The model under review builds one solid part; all positions refer to its coordinate system, in mm. A direction names the side the tool comes from. Coordinates: 2 decimals unless noted, no trailing zeros. Order: outer loops, then holes, each group sorted by start corner. A loop starts at its lowest first (then second) coordinate and runs counter-clockwise, first axis right, second up. Notation, with made-up numbers: M 40.5,58 L 83.5,58 A14 cw 83.5,75 Z; hole C 21.25,10.5 d9. An arc over 180 degrees is marked long. Answer as CSV lines item,"result". Start each with the question number.
Q1. Machinability: for faces 4 (the face through (19.48, 9.86, 19.41)), 5 (the face through (-16.754, 4.93, 50.282)), 6 (the face through (18, 5, 53)), 7 (the face through (9, 15, 40)), 8 (the face through (-51.03, 4.93, -11.14)), which of the approach directions +Z, -Z, +X, -X, +Y, -Y give a long, thin tool a straight path to every point of the face, cutting with its end or side? Answer none if there is none.
Q2. Consider section B-B on z = 9. Write out the cut boundary in (x, y).
Q3. The part is to be moulded in two halves that separate along Z. For faces 1 (the face through (43.39, 4.93, -49.58)), 2 (the face through (-56.438, 4.93, 47.596)), 3 (the face through (27.737, 9.86, 15.957)), say which applies: +Z half, -Z half, draft (parallel to the pull), parting line (faces both ways), or undercut.
Q4. Wall thickness on L1, parallel to Z at x = 35, y = 8.25; L2, parallel to Z at x = 9.5, y = 4; L3, parallel to Y at x = -41, z = 38: over which ranges is each line inside the solid? List them lowest first. Write a range as [from, to].
Q5. For P1, Ø2.5, axis at y = 13.5, z = -30.5, coming from the -X side; P2, Ø2.5, axis at y = 10.5, z = -30, coming from the +X side; P3, Ø10, axis at x = -36, z = -30, coming from the +Y side; P4, Ø3.5, axis at y = 12, z = 30.5, coming from the -X side, all flat-tipped, find the tip position at first contact; note any pin that passes through.
Q6. Consider section A-A on x = -65. Write out the cut boundary in (y, z).
Q7. Consider section C-C on z = -23.5. Write out the cut boundary in (x, y), and give its area (3 significant figures).
Autodesk Inventor part; units mm, degrees
ref_plane "YZ Plane" through (0, 0, 0) normal (1, 0, 0) x (0, 1, 0)
ref_plane "XZ Plane" through (0, 0, 0) normal (0, 1, 0) x (-1, 0, 0)
ref_plane "XY Plane" through (0, 0, 0) normal (0, 0, 1) x (1, 0, 0)
sketch "Sketch1" plane through (0, 0, 0) normal (0, 1, 0) x (-1, 0, 0)
  circle A0 centre (0, 0) radius 41
  line L0 (-47, 0) -> (-47, 41)
  line L1 (-35, 53) -> (0, 53)
  circle A1 centre (-35, 41) radius 6
  arc A2 (-35, 53) -> (-47, 41) centre (-35, 41) ccw
  circle A3 centre (73.6122, 42.5) radius 6
  circle A4 centre (56.2917, 32.5) radius 6
  line L2 (0, 0) -> (41, 0) construction
  line L3 (0, 0) -> (35.507, 20.5) construction
  line L4 (35.507, 20.5) -> (56.2917, 32.5) construction
  line L5 (56.2917, 32.5) -> (73.6122, 42.5) construction
  arc A5 (80.1122, 31.2417) -> (67.1122, 53.7583) centre (73.6122, 42.5) ccw
  line L6 (67.1122, 53.7583) -> (45.4615, 41.2583)
  line L7 (80.1122, 31.2417) -> (59, 19.0526)
  arc A6 (59, 19.0526) -> (48, 0) centre (70, 0) ccw
  arc A7 (32.1763, 42.1151) -> (45.4615, 41.2583) centre (39.4615, 51.6506) ccw
  line L8 (41, 0) -> (48, 0) construction
  circle A8 centre (73.6122, -42.5) radius 6
  circle A9 centre (56.2917, -32.5) radius 6
  arc A10 (67.1122, -53.7583) -> (80.1122, -31.2417) centre (73.6122, -42.5) ccw
  line L9 (67.1122, -53.7583) -> (45.4615, -41.2583)
  line L10 (80.1122, -31.2417) -> (59, -19.0526)
  arc A11 (48, 0) -> (59, -19.0526) centre (70, 0) ccw
  arc A12 (45.4615, -41.2583) -> (32.1763, -42.1151) centre (39.4615, -51.6506) ccw
  arc A13 (3.5, 31.808) -> (-3.5, 31.808) centre (0, 0) ccw
  arc A14 (10.6071, 25.372) -> (3.5, 27.2764) centre (0, 0) ccw
  line L11 (3.5, 31.808) -> (3.5, 27.2764)
  arc A15 (-12.8729, 29.2966) -> (-18.9351, 25.7966) centre (0, 0) ccw
  line L12 (-12.8729, 29.2966) -> (-10.6071, 25.372)
  arc A16 (-25.7966, 18.9351) -> (-29.2966, 12.8729) centre (0, 0) ccw
  line L13 (-25.7966, 18.9351) -> (-21.872, 16.6693)
  arc A17 (-31.808, 3.5) -> (-31.808, -3.5) centre (0, 0) ccw
  line L14 (-31.808, 3.5) -> (-27.2764, 3.5)
  arc A18 (-29.2966, -12.8729) -> (-25.7966, -18.9351) centre (0, 0) ccw
  line L15 (-29.2966, -12.8729) -> (-25.372, -10.6071)
  arc A19 (-18.9351, -25.7966) -> (-12.8729, -29.2966) centre (0, 0) ccw
  line L16 (-18.9351, -25.7966) -> (-16.6693, -21.872)
  arc A20 (-3.5, -31.808) -> (3.5, -31.808) centre (0, 0) ccw
  line L17 (-3.5, -31.808) -> (-3.5, -27.2764)
  arc A21 (12.8729, -29.2966) -> (18.9351, -25.7966) centre (0, 0) ccw
  line L18 (12.8729, -29.2966) -> (10.6071, -25.372)
  arc A22 (25.7966, -18.9351) -> (29.2966, -12.8729) centre (0, 0) ccw
  line L19 (25.7966, -18.9351) -> (21.872, -16.6693)
  arc A23 (31.808, -3.5) -> (31.808, 3.5) centre (0, 0) ccw
  line L20 (31.808, -3.5) -> (27.2764, -3.5)
  arc A24 (29.2966, 12.8729) -> (25.7966, 18.9351) centre (0, 0) ccw
  line L21 (29.2966, 12.8729) -> (25.372, 10.6071)
  arc A25 (18.9351, 25.7966) -> (12.8729, 29.2966) centre (0, 0) ccw
  line L22 (18.9351, 25.7966) -> (16.6693, 21.872)
  line L23 (10.6071, 25.372) -> (12.8729, 29.2966)
  arc A26 (-3.5, 27.2764) -> (-10.6071, 25.372) centre (0, 0) ccw
  line L24 (-3.5, 27.2764) -> (-3.5, 31.808)
  arc A27 (-16.6693, 21.872) -> (-21.872, 16.6693) centre (0, 0) ccw
  line L25 (-16.6693, 21.872) -> (-18.9351, 25.7966)
  arc A28 (-25.372, 10.6071) -> (-27.2764, 3.5) centre (0, 0) ccw
  line L26 (-25.372, 10.6071) -> (-29.2966, 12.8729)
  arc A29 (-27.2764, -3.5) -> (-25.372, -10.6071) centre (0, 0) ccw
  line L27 (-27.2764, -3.5) -> (-31.808, -3.5)
  arc A30 (-21.872, -16.6693) -> (-16.6693, -21.872) centre (0, 0) ccw
  line L28 (-21.872, -16.6693) -> (-25.7966, -18.9351)
  arc A31 (-10.6071, -25.372) -> (-3.5, -27.2764) centre (0, 0) ccw
  line L29 (-10.6071, -25.372) -> (-12.8729, -29.2966)
  arc A32 (3.5, -27.2764) -> (10.6071, -25.372) centre (0, 0) ccw
  line L30 (3.5, -27.2764) -> (3.5, -31.808)
  arc A33 (16.6693, -21.872) -> (21.872, -16.6693) centre (0, 0) ccw
  line L31 (16.6693, -21.872) -> (18.9351, -25.7966)
  arc A34 (25.372, -10.6071) -> (27.2764, -3.5) centre (0, 0) ccw
  line L32 (25.372, -10.6071) -> (29.2966, -12.8729)
  arc A35 (27.2764, 3.5) -> (25.372, 10.6071) centre (0, 0) ccw
  line L33 (27.2764, 3.5) -> (31.808, 3.5)
  arc A36 (21.872, 16.6693) -> (16.6693, 21.872) centre (0, 0) ccw
  line L34 (21.872, 16.6693) -> (25.7966, 18.9351)
  line L35 (-47, 0) -> (-47, -41)
  line L36 (-35, -53) -> (0, -53)
  circle A37 centre (-35, -41) radius 6
  arc A38 (-47, -41) -> (-35, -53) centre (-35, -41) ccw
  arc A39 (32.1763, 42.1151) -> (0, 53) centre (0, 0) ccw
  arc A40 (0, -53) -> (32.1763, -42.1151) centre (0, 0) ccw
  point P0 (25.7966, 18.9351)
  point P1 (31.808, 3.5)
  point P2 (29.2966, -12.8729)
  point P3 (18.9351, -25.7966)
  point P4 (3.5, -31.808)
  point P5 (-12.8729, -29.2966)
  point P6 (-25.7966, -18.9351)
  point P7 (-31.808, -3.5)
  point P8 (-29.2966, 12.8729)
  point P9 (-3.5, 31.808)
  dimension "d0" = 82
  dimension "d1" = 12
  dimension "d2" = 12
  dimension "d3" = 35
  dimension "d4" = 41
  dimension "d7" = 30
  dimension "d8" = 24
  dimension "d9" = 20
  dimension "d10" = 13
  dimension "d11" = 22
  dimension "d12" = 12
  dimension "d14" = 64
  dimension "d15" = 55
  dimension "d16" = 7
  dimension "d19" = 360
  dimension "d23" = 360
  dimension "d25" = 53
extrude "Extrusion1" add sketch "Sketch1" along normal blind 10 contours L0 A2 L1 A39 A7 L6 A5 L7 A6 A11 L10 A10 L9 A12 A40 L36 A38 L35
extrude "Extrusion2" add sketch "Sketch1" along normal blind 20 contours A0
properties part number "Splined_Flange_Mount"
Evaluation:
1,face 4,"+Y, -Y"
1,face 5,"+Z, +Y, -Y"
1,face 6,"+Z, +X, +Y, -Y"
1,face 7,"+Y"
1,face 8,"-X, +Y, -Y"
2,outline,"M -49.93,0 L -25.99,0 L -25.99,20 L -40,20 L -40,10 L -49.93,10 Z; M 25.99,0 L 47,0 L 47,10 L 40,10 L 40,20 L 25.99,20 Z"
3,face 1,"-Z half"
3,face 2,"+Z half"
3,face 3,"undercut"
4,L1,"z = [-53, -47], [-35, 35], [47, 53]"
4,L2,"z = [-53, -25.81], [25.81, 53]"
4,L3,"y = [0, 10]"
5,P1,"stops at x = -28.73"
5,P2,"stops at x = 47"
5,P3,"stops at y = 10"
5,P4,"stops at x = -29.23"
6,outline,"M 0,-52.54 L 10,-52.54 L 10,-22.52 L 0,-22.52 Z; M 0,22.52 L 10,22.52 L 10,52.54 L 0,52.54 Z"
7,outline,"M -66.7,0 L -17.61,0 L -17.61,20 L -33.6,20 L -33.6,10 L -66.7,10 Z; M 17.61,0 L 47,0 L 47,10 L 33.6,10 L 33.6,20 L 17.61,20 Z"
7,area,"1,100 mm²"
